Build history of the part. All positions in model axes, mm. A direction names the side the tool comes from. Round coordinates to 2 decimals unless told otherwise and drop trailing zeros. Write each loop counter-clockwise with the first axis right and the second up, starting at its lowest first coordinate (ties: lowest second). Pieces come first, ordered by that corner, then holes. Notation, with made-up numbers: (26.5, -19.5) - (67.5, -19.5) arc R30 cw to (67.5, 12.5) - close; hole circle Ø4 at (46.25, 26.25). An arc over 180 degrees is marked (long way). Answer as a JSON object with one key per item and string values. Group by question number.
Item 1: Two-plate mould, pull along X, no slides. Class faces 5 (the cylindrical face through (1, -0.32, -8.11)), 6 (the cylindrical face through (-0.54, 2.44, -2.78)), 7 (the flat face through (0, 3, -6)): +X half, -X half, draft (parallel to the pull), parting line (faces both ways), or undercut.
Item 2: Slice it at C-C, the plane z = -10. List the corners of the cut face in (x, y).
Item 3: Which spindle directions (+Z, -Z, +X, -X, +Y, -Y) get a long thin tool onto all of the face, cutting with end or side? Do faces 1 (the cylindrical face through (2.003, -0.631, -9.521)), 2 (the cylindrical face through (2.003, -0.631, -15.254)), 3 (the flat face through (-3, 0, -5)), 4 (the flat face through (1, -1, 0)). Say none if no direction does.
Item 4: Slice it at B-B, the plane z = -7.5. List the corners of the cut face in (x, y), then the cut area to 3 significant figures.
Item 5: Slice it at D-D, the plane z = -12.75. List the corners of the cut face in (x, y), then the cut area to 3 significant figures.
Item 6: Flat gauge pins, fed straight in: pin 1 (2 mm diameter, centred on x = -1.5, z = -14, fed in from -Y); pin 2 (2 mm diameter, centred on y = -1, z = -2.5, fed in from +X); pin 3 (2 mm diameter, centred on y = -2, z = -5.5, fed in from +X). Where does each tip first touch, or does it go through?
Item 7: Probe line 1 (Y direction, x = 0, z = -8.25); line 2 (Y direction, x = 0, z = -7.75); line 3 (Z direction, x = -2.75, y = 0.75). List the from-to ranges inside material, lowest first. Write a range as from..to.
Item 8: Slice it at A-A, the plane x = 0. List the corners of the cut face in (y, z), then the cut area to 3 significant figures.
Autodesk Inventor part; units mm, degrees
ref_plane "YZ Plane" through (0, 0, 0) normal (1, 0, 0) x (0, 1, 0)
ref_plane "XZ Plane" through (0, 0, 0) normal (0, 1, 0) x (-1, 0, 0)
ref_plane "XY Plane" through (0, 0, 0) normal (0, 0, 1) x (1, 0, 0)
sketch "Sketch1" plane through (0, 0, 0) normal (0, 1, 0) x (-1, 0, 0)
  line L0 (-1.05, 0) -> (-2.5, 0)
  line L1 (-2.5, 0) -> (-2.5, -5)
  line L2 (-2.5, -5) -> (-2.1, -5)
  line L3 (-2.1, -5) -> (-2.1, -16)
  line L4 (-2.1, -16) -> (-1.05, -16)
  line L5 (0, -19.2) -> (0, 3.2)
  line L6 (-1.05, 0) -> (-1.05, -16)
  line L7 (-2.1, -11) -> (-2.65, -11)
  line L8 (-2.65, -11) -> (-2.1, -15)
  point P0 (0, 0)
  dimension "d0" = 11
  dimension "d1" = 5
  dimension "d3" = 1.05
  dimension "d4" = 2.5
  dimension "d14" = 2.1
  dimension "d15" = 2.65
  dimension "d19" = 1
  dimension "d20" = 4
revolve "Revolution1" add sketch "Sketch1" angle 360 about axis through (0, 0, -10) along (0, 0, 1)
fillet "Fillet2" radius 0.5 2 edges at (-2.5, 0, 0) (-2.1, 0, -16)
sketch "Sketch3" plane through (0, 0, -5) normal (0, 0, -1) x (-1, 0, 0)
  line L0 (3.4641, 0) -> (1.7321, -3)
  line L1 (1.7321, -3) -> (-1.7321, -3)
  line L2 (-1.7321, -3) -> (-3.4641, 0)
  line L3 (-3.4641, 0) -> (-1.7321, 3)
  line L4 (-1.7321, 3) -> (1.7321, 3)
  line L5 (1.7321, 3) -> (3.4641, 0)
  circle A0 centre (0, 0) radius 1.05
  dimension "d21" = 6
extrude "Extrusion2" add sketch "Sketch3" along normal blind 3
properties part number "Suction_electrode_cap_side_dk"
Geometry says:
{
 "1": {"face 5": "undercut", "face 6": "parting line", "face 7": "draft"},
 "2": {"outline": "circle Ø4.2 at (0, 0); hole circle Ø2.1 at (0, 0)"},
 "3": {"face 1": "none", "face 2": "-Z", "face 3": "+Z", "face 4": "+Z, +X, -X, +Y, -Y"},
 "4": {"outline": "(-3.46, 0) - (-1.73, -3) - (1.73, -3) - (3.46, 0) - (1.73, 3) - (-1.73, 3) - close; hole circle Ø2.1 at (0, 0)", "area": "27.7 mm^2"},
 "5": {"outline": "circle Ø4.82 at (0, 0); hole circle Ø2.1 at (0, 0)", "area": "14.8 mm^2"},
 "6": {"pin 1": "stops at y = -2.22", "pin 2": "stops at x = 2.5", "pin 3": "stops at x = 2.89"},
 "7": {"line 1": "y = -2.1..-1.05, 1.05..2.1", "line 2": "y = -3..-1.05, 1.05..3", "line 3": "z = -8..-5"},
 "8": {"outline": "(-3, -8) - (-2.1, -8) - (-2.1, -11) - (-2.65, -11) - (-2.1, -15) - (-2.1, -15.5) arc R0.5 ccw to (-1.6, -16) - (-1.05, -16) - (-1.05, 0) - (-2, 0) arc R0.5 ccw to (-2.5, -0.5) - (-2.5, -5) - (-3, -5) - close; (1.05, -16) - (1.6, -16) arc R0.5 ccw to (2.1, -15.5) - (2.1, -15) - (2.65, -11) - (2.1, -11) - (2.1, -8) - (3, -8) - (3, -5) - (2.5, -5) - (2.5, -0.5) arc R0.5 ccw to (2, 0) - (1.05, 0) - close", "area": "45.0 mm^2"}
}
